Could you check a few things on this model? Use its own coordinates, in mm. Round coordinates to 2 decimals unless told otherwise and drop trailing zeros. Loops run counter-clockwise (first coordinate to the right, second up) from the corner with the lowest first, then second, coordinate; pieces in that order, holes last. Notation, with made-up numbers: (57, -9) -> (98, -9) arc R29 cw to (98, 15) -> close; hole circle Ø9 at (-31.5, 15.25). An arc over 180 degrees is marked (long way). Use CSV: the item, a comma, the result in double quotes. Start each with the question number.
```python
from build123d import *

# Parameters (mm, degrees)
EXTRUDE_1_DEPTH              = 4
FILLET_1_R                   = 2
HOLE_WIZARD_M4_1_D           = 4.5
HOLE_WIZARD_M4_1_DEPTH       = 24.5
HOLE_WIZARD_M4_1_CSINK_D     = 9.18
HOLE_WIZARD_M4_1_CSINK_ANGLE = 90
HOLE_WIZARD_M4_1_TIP         = 1.351936393
HOLE_WIZARD_M3_1_D           = 3.4
HOLE_WIZARD_M3_1_DEPTH       = 24.5
HOLE_WIZARD_M3_1_CSINK_D     = 6.94
HOLE_WIZARD_M3_1_CSINK_ANGLE = 90
HOLE_WIZARD_M3_1_TIP         = 1.021463052
EXTRUDE_2_DEPTH              = 4
FILLET_2_R                   = 3


with BuildPart() as part:
    # 草图1 → 凸台-拉伸1 (new body)
    with BuildSketch(Plane.XY):
        Polygon((0, 0), (-15, 0), (-15, 26.213203436), (20, 61.213203436), (20, 81.213203436), (35, 81.213203436), (35, 55), (0, 20), align=None)
    extrude(amount=EXTRUDE_1_DEPTH)

    # 圆角1
    fillet_1_edges = [part.edges().sort_by_distance(p)[0] for p in [
        (0, 0, 2),
        (-15, 0, 2),
        (-15, 26.213203436, 2),
        (20, 61.213203436, 2),
        (20, 81.213203436, 2),
        (35, 81.213203436, 2),
        (35, 55, 2),
        (0, 20, 2),
    ]]
    fillet(fillet_1_edges, radius=FILLET_1_R)

    # M4 六角凹锥坑头螺钉的锥形沉头孔1
    with Locations(Plane(origin=(27.5, 76.213203436, 4), x_dir=(1, 0, 0), z_dir=(0, 0, 1))):
        with Locations((0, 0), (0, -10), (-35, -61.213203436), (-35, -71.213203436)):
            CounterSinkHole(HOLE_WIZARD_M4_1_D / 2, HOLE_WIZARD_M4_1_CSINK_D / 2, depth=HOLE_WIZARD_M4_1_DEPTH, counter_sink_angle=HOLE_WIZARD_M4_1_CSINK_ANGLE)
            with Locations((0, 0, -(HOLE_WIZARD_M4_1_DEPTH + HOLE_WIZARD_M4_1_TIP / 2))):  # 118° drill point
                Cone(0, HOLE_WIZARD_M4_1_D / 2, HOLE_WIZARD_M4_1_TIP, mode=Mode.SUBTRACT)

    # M3 六角凹锥坑头螺钉的锥形沉头孔1
    with Locations(Plane(origin=(4.343145751, 34.949747468, 4), x_dir=(1, 0, 0), z_dir=(0, 0, 1))):
        with Locations((0, 0), (11.313708498, 11.313708499)):
            CounterSinkHole(HOLE_WIZARD_M3_1_D / 2, HOLE_WIZARD_M3_1_CSINK_D / 2, depth=HOLE_WIZARD_M3_1_DEPTH, counter_sink_angle=HOLE_WIZARD_M3_1_CSINK_ANGLE)
            with Locations((0, 0, -(HOLE_WIZARD_M3_1_DEPTH + HOLE_WIZARD_M3_1_TIP / 2))):  # 118° drill point
                Cone(0, HOLE_WIZARD_M3_1_D / 2, HOLE_WIZARD_M3_1_TIP, mode=Mode.SUBTRACT)

    # 草图6 → 凸台-拉伸2 (add)
    with BuildSketch(Plane.XY.offset(4)):
        with BuildLine():
            Line((34.414213562, 54.414213562), (50, 70))
            Line((50, 70), (50, 81.213203436))
            Line((50, 81.213203436), (33, 81.213203436))
            ThreePointArc((33, 81.213203436), (34.414213562, 80.627416998), (35, 79.213203436))
            Line((35, 79.213203436), (35, 55.828427125))
            ThreePointArc((35, 55.828427125), (34.847759065, 55.06306026), (34.414213562, 54.414213562))
        make_face()
    extrude(amount=-EXTRUDE_2_DEPTH)

    # 圆角2
    fillet_2_edges = [part.edges().sort_by_distance(p)[0] for p in [
        (50, 70, 2),
        (50, 81.213203436, 2),
    ]]
    fillet(fillet_2_edges, radius=FILLET_2_R)


solid = part.part
```
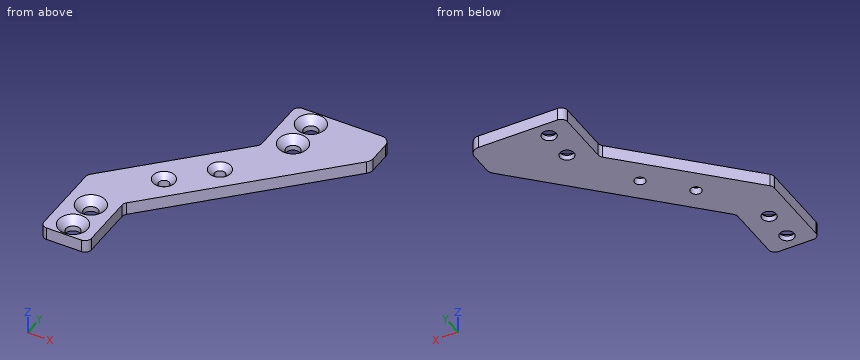
1. Suppose I cut it at D-D (x = 40). List the corners of the cut face in (y, z) for me, then the cut area to 3 significant figures.
2. If I drill on L1, parallel to X at y = 5, z = 1.35; L2, parallel to Y at x = 25, z = 3.05; L3, parallel to X at y = 71.5, z = 2.3, over which ranges is the centre line in solid material (lowest first)?
3. Suppose I cut it at C-C (z = 0.6). List the corners of the cut face in (x, y) for me.
4. Will these pins go through, and if not, where does the flat tip stop? pin 1 (2.5 mm diameter, centred on x = 15.66, y = 46.26, fed in from -Z); pin 2 (1.5 mm diameter, centred on x = 41, z = 1, fed in from -Y); pin 3 (7 mm diameter, centred on x = -7.5, y = 5, fed in from +Z); pin 4 (6 mm diameter, centred on x = 27.5, y = 76.21, fed in from +Z).
5. Suppose I cut it at B-B (y = 5). List the corners of the cut face in (x, z) for me, then the cut area to 3 significant figures.
6. Suppose I cut it at A-A (x = 27.5). List the corners of the cut face in (y, z) for me.
Geometry check:
1,outline,"(60, 0) -> (81.21, 0) -> (81.21, 4) -> (60, 4) -> close"
1,area,"84.9 mm²"
2,L1,"x = -15 to -9.75, -5.25 to 0"
2,L2,"y = 45 to 63.57, 68.86 to 73.57, 78.86 to 81.21"
2,L3,"x = 20 to 50"
3,outline,"(-15, 2) arc R2 ccw to (-13, 0) -> (-2, 0) arc R2 ccw to (0, 2) -> (0, 19.17) arc R2 cw to (0.59, 20.59) -> (49.12, 69.12) arc R3 ccw to (50, 71.24) -> (50, 78.21) arc R3 ccw to (47, 81.21) -> (22, 81.21) arc R2 ccw to (20, 79.21) -> (20, 62.04) arc R2 cw to (19.41, 60.63) -> (-14.41, 26.8) arc R2 ccw to (-15, 25.38) -> close; hole circle Ø4.5 at (-7.5, 5); hole circle Ø4.5 at (-7.5, 15); hole circle Ø3.4 at (4.34, 34.95); hole circle Ø3.4 at (15.66, 46.26); hole circle Ø4.5 at (27.5, 66.21); hole circle Ø4.5 at (27.5, 76.21)"
4,pin 1,"passes through"
4,pin 2,"stops at y = 60.25"
4,pin 3,"stops at z = 2.91"
4,pin 4,"stops at z = 2.41"
5,outline,"(-15, 0) -> (-9.75, 0) -> (-9.75, 1.66) -> (-12.09, 4) -> (-15, 4) -> close; (-5.25, 0) -> (0, 0) -> (0, 4) -> (-2.91, 4) -> (-5.25, 1.66) -> close"
5,area,"36.5 mm²"
6,outline,"(47.5, 0) -> (63.96, 0) -> (63.96, 1.66) -> (61.62, 4) -> (47.5, 4) -> close; (68.46, 0) -> (73.96, 0) -> (73.96, 1.66) -> (71.62, 4) -> (70.8, 4) -> (68.46, 1.66) -> close; (78.46, 0) -> (81.21, 0) -> (81.21, 4) -> (80.8, 4) -> (78.46, 1.66) -> close"
